Drawing for the job (mm, zero at the part's lowest x, y, z). A direction names the side the tool comes from. Coordinates: 2 decimals unless noted, no trailing zeros. Order: outer loops, then holes, each group sorted by start corner. A loop starts at its lowest first (then second) coordinate and runs counter-clockwise, first axis right, second up. Notation, with made-up numbers: (4, -35.5) -> (32, -35.5) arc R16 cw to (32, -11.5) -> close; hole circle Ø6 at (80, -10.5). An arc over 180 degrees is marked (long way). Write each question's results on one line, items separated by ' | '.
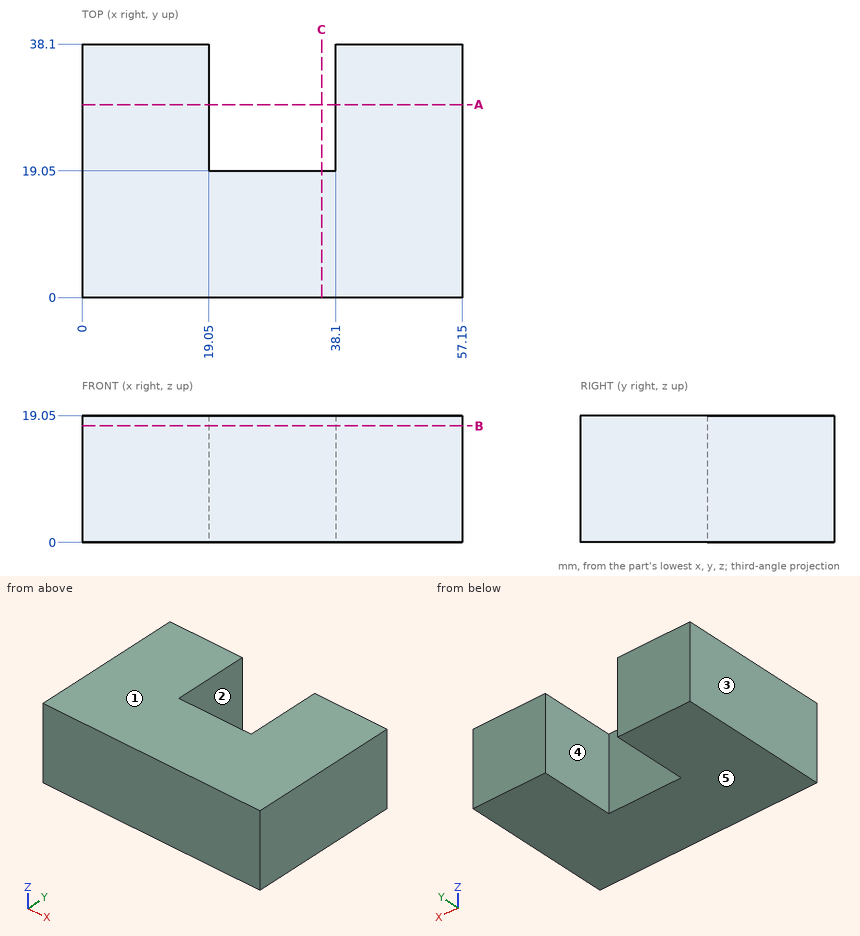
Item 1: Pull direction X, two halves, no side cores. Call the marked faces 1, 2 and 3: released by +X, released by -X, zero draft, split by the parting line, or undercut.
Answer:
face 1: zero draft | face 2: undercut | face 3: released by -X
Item 2: Tool access for the marked faces 4 and 5: list every direction of +Z, -Z, +X, -X, +Y, -Y with a clear straight run to the whole face (end or side of a thin tool).
Answer:
face 4: +Z, -Z, +Y | face 5: -Z, +X, -X, +Y, -Y
Item 3: Drill centre lines: line 1 (X direction, y = 32.5, z = 18); line 2 (Y direction, x = 19.5, z = 15). Where is each one in solid material? Low to high. Write a range as from..to.
Answer:
line 1: x = 0..19.05, 38.1..57.15 | line 2: y = 0..19.05
Item 4: Slice it at C-C, the plane x = 36. List the corners of the cut face in (y, z).
Answer:
outline: (0, 0) -> (19.05, 0) -> (19.05, 19.05) -> (0, 19.05) -> close
Item 5: Pin check, flat tip, straight feed: pin 1 (5.5 mm diameter, centred on x = 30.5, z = 7.5, fed in from +Y). Stop position of the tip, or through.
Answer:
pin 1: stops at y = 19.05
Item 6: Slice it at A-A, the plane y = 29. List the corners of the cut face in (x, z), and give its area (3 significant figures).
Answer:
outline: (0, 0) -> (19.05, 0) -> (19.05, 19.05) -> (0, 19.05) -> close; (38.1, 0) -> (57.15, 0) -> (57.15, 19.05) -> (38.1, 19.05) -> close | area: 726 mm^2
Item 7: Slice it at B-B, the plane z = 17.5. List the corners of the cut face in (x, y), and give its area (3 significant figures).
Answer:
outline: (0, 0) -> (57.15, 0) -> (57.15, 38.1) -> (38.1, 38.1) -> (38.1, 19.05) -> (19.05, 19.05) -> (19.05, 38.1) -> (0, 38.1) -> close | area: 1,810 mm^2
